The listing builds one solid part. Answer for the finished solid, in the listing's coordinates (mm). A direction names the side the tool comes from. Give positions to 0.01 mm unless a question says otherwise; leave off trailing zeros. Order: outer loops, then holes, each group sorted by start corner. A loop starts at its lowest first (then second) coordinate and runs counter-clockwise, first axis right, second up. Notation, with made-up numbers: (-39.5, 28) - (2.5, 28) arc R9 ccw to (2.5, 38) - close; hole circle Ø5 at (31.5, 11). An arc over 180 degrees is marked (long way). Write each question's results on one line, items separated by ' | '. Start each with the question number.
1. Section D-D (z = -41) is taken. Give the vertices of the cut face in (x, y), and give its area (3 significant figures).
2. Section A-A (x = 149) is taken. Give the vertices of the cut face in (y, z).
3. Find the intervals of material crossed by L1, parallel to Z at x = 164, y = 46.5; L2, parallel to Z at x = 93, y = 121.5; L3, parallel to X at y = 80.5, z = -26.5, in increasing order.
4. Which of the six approach directions +Z, -Z, +X, -X, +Y, -Y give full straight-line access (tool end or side, diameter ignored) to faces 4 (the face through (125, 181.939, -4)), 5 (the face through (125, 131.139, 48)), 6 (the face through (125, 157, 73.136)), 7 (the face through (-11.59, 50.09, 115.74)), 8 (the face through (12.7, 50, 81))?
5. Section B-B (y = 96.5) is taken. Give the vertices of the cut face in (x, z), and give its area (3 significant figures).
6. Section C-C (z = 33) is taken. Give the vertices of the cut face in (x, y), and give its area (3 significant figures).
7. Flat-ended cylindrical pins translate along their axes: pin 1 (4 mm diameter, centred on y = 160, z = 57.5, fed in from -X); pin 2 (1.5 mm diameter, centred on x = 156.5, y = 97.5, fed in from +Z). Find the tip coordinate at first contact, or state that the pin passes through.
8. Determine the mould class of faces 1 (the face through (109, 39, 0)), 2 (the face through (125, 80.339, -39)), 3 (the face through (107, 101.6, 50)) for opening direction Y: released by +Y, released by -Y, zero draft, split by the parting line, or undercut.
from build123d import *

# Parameters (mm, degrees)
F1_DEPTH = 101.6
F3_DEPTH = 254


with BuildPart() as f1:
    # F0 (on Front) → F1 (new body)
    with BuildSketch(Plane.XZ):
        Polygon((-31.363741, 0), (0, 0), (254, 0), (254, 127), (203.2, 127), (203.2, 50.8), (12.7, 50.8), (12.7, 112.531804), (-36.5729, 119.043261), align=None)
    extrude(amount=-F1_DEPTH)

    # F2 (on Right) → F3 (join)
    with BuildSketch(Plane.YZ):
        Polygon((80.338995, 22.33608), (80.338995, -79.26392), (181.938995, -79.26392), (181.938995, 73.13608), (131.138995, 73.13608), (131.138995, 22.33608), align=None)
    extrude(amount=F3_DEPTH)


solid = f1.part
Reported:
1) outline: (0, 80.34) - (254, 80.34) - (254, 181.94) - (0, 181.94) - close | area: 25,800 mm²
2) outline: (0, 0) - (80.34, 0) - (80.34, -79.26) - (181.94, -79.26) - (181.94, 73.14) - (131.14, 73.14) - (131.14, 22.34) - (101.6, 22.34) - (101.6, 50.8) - (0, 50.8) - close
3) L1: 0 to 50.8 | L2: -79.26 to 22.34 | L3: 0 to 254
4) face 4: +Z, -Z, +X, -X, +Y | face 5: +Z, +X, -X | face 6: +Z, +X, -X, +Y | face 7: +Z, +Y, -Y | face 8: +Z, -Y
5) outline: (-36.57, 119.04) - (-31.36, 0) - (0, 0) - (0, -79.26) - (254, -79.26) - (254, 127) - (203.2, 127) - (203.2, 50.8) - (12.7, 50.8) - (12.7, 112.53) - close | area: 41,700 mm²
6) outline: (-32.81, 0) - (254, 0) - (254, 101.6) - (-32.81, 101.6) - close; (0, 131.14) - (254, 131.14) - (254, 181.94) - (0, 181.94) - close | area: 42,000 mm²
7) pin 1: x = 0 | pin 2: z = 50.8
8) face 1: zero draft | face 2: released by -Y | face 3: undercut
